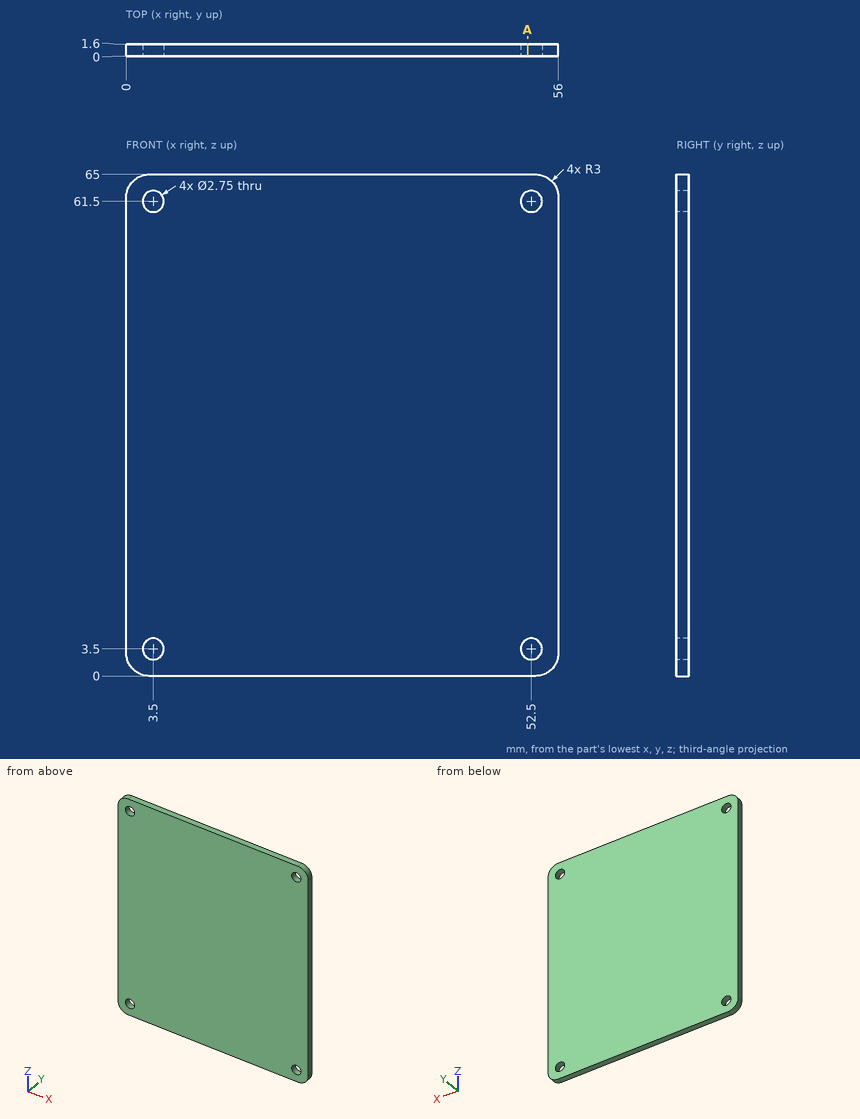
Study the drawing (mm; zero at the part's minimum x, y, z) and answer. Give positions to 0.01 mm unless a question says otherwise; leave off trailing zeros. Write each loop counter-clockwise with the first axis right and the second up, starting at its lowest first coordinate (ties: lowest second). Pieces come first, ordered by that corner, then holes.
(1) Straight lines are drawn through the part: line 1 (Z direction, x = 52.5, y = 0.7) (3 decimals); line 2 (X direction, y = 0.9, z = 3.5) (3 decimals); line 3 (Z direction, x = 53.5, y = 1.05) (1 decimal). For each, find the intervals that lie inside material, in ascending order.
Final values:
line 1: z = 0 to 2.125, 4.875 to 60.125, 62.875 to 65
line 2: x = 0 to 2.125, 4.875 to 51.125, 53.875 to 56
line 3: z = 0 to 2.6, 4.4 to 60.6, 62.4 to 65
(2) The part is cut by section A-A on x = 52. Write down the section's boundary in (y, z).
Final values:
outline: (0, 0) - (1.6, 0) - (1.6, 2.22) - (0, 2.22) - close; (0, 4.78) - (1.6, 4.78) - (1.6, 60.22) - (0, 60.22) - close; (0, 62.78) - (1.6, 62.78) - (1.6, 65) - (0, 65) - close
(3) A flat-ended cylindrical pin translates along its axis: pin 1 Ø2 at (x, z) = (3.5, 3.5) entering from -Y. Find the tip coordinate at first contact, or state that the pin passes through.
Final values:
pin 1: passes through
